```python
from build123d import *

# Parameters (mm, degrees)
F0_W     = 10
F0_H     = 4
F0_R     = 0.4
F0_R_2   = 0.425
F0_R_3   = 0.45
F0_R_4   = 0.475
F0_R_5   = 0.5
F1_DEPTH = 3
F2_R     = 1


with BuildPart() as f1:
    # F0 (on Front) → F1 (new body)
    with BuildSketch(Plane.XZ):
        Rectangle(F0_W, F0_H)
        with Locations((-3.333333, 0)):
            Circle(F0_R, mode=Mode.SUBTRACT)
        with Locations((-1.666667, 0)):
            Circle(F0_R_2, mode=Mode.SUBTRACT)
        Circle(F0_R_3, mode=Mode.SUBTRACT)
        with Locations((1.666667, 0)):
            Circle(F0_R_4, mode=Mode.SUBTRACT)
        with Locations((3.333333, 0)):
            Circle(F0_R_5, mode=Mode.SUBTRACT)
    extrude(amount=F1_DEPTH)

    # F2
    f2_edges = [f1.edges().sort_by_distance(p)[0] for p in [
        (5, -1.5, 2),
        (5, -1.5, -2),
    ]]
    fillet(f2_edges, radius=F2_R)


solid = f1.part
```
Geometry check sheet. Reference: the model listing, model coordinates, mm. Coordinates: 2 decimals unless noted, no trailing zeros. Write each loop counter-clockwise with the first axis right and the second up, starting at its lowest first coordinate (ties: lowest second). Pieces come first, ordered by that corner, then holes. Notation, with made-up numbers: M 41.25,16.25 L 89.25,16.25 A29 ccw 89.25,42.25 Z; hole C -31.75,22.25 d6. An arc over 180 degrees is marked long. Use one line per item in the form item = value. Start each with the question number.
1) Section check A-A on z = 0. Enter the section's corners in (x, y).
2) Section check D-D on x = 1.5. Enter the section's corners in (y, z).
3) Section check B-B on x = 0. Enter the section's corners in (y, z).
4) Release check for a two-part mould opening along Z. For faces 1 (the cylindrical face through (4.699, -1.521, -1.715)), 2 (the flat face through (-1, -1, 2)), 3 (the flat face through (0, -3, 1)), 4 (the cylindrical face through (3.795, -1.479, -0.192)) record: pulls with the +Z half, pulls with the -Z half, needs draft (parallel to the pull), parting line crosses it, or undercut.
5) Thickness scan on probe 1 along Z at (x, y) = (0, -0.7); probe 2 along X at (y, z) = (-0.65, -0.15); probe 3 along Z at (x, y) = (2, -2). Record the ranges inside material, lowest first. Write a range as from..to.
6) Section check C-C on y = -2.5. Enter the section's corners in (x, z) (3 decimals), and give its area (3 significant figures).
Responses:
q1.outline = M -5,-3 L -3.73,-3 L -3.73,0 L -5,0 Z; M -2.93,-3 L -2.09,-3 L -2.09,0 L -2.93,0 Z; M -1.24,-3 L -0.45,-3 L -0.45,0 L -1.24,0 Z; M 0.45,-3 L 1.19,-3 L 1.19,0 L 0.45,0 Z; M 2.14,-3 L 2.83,-3 L 2.83,0 L 2.14,0 Z; M 3.83,-3 L 5,-3 L 5,0 L 3.83,0 Z
q2.outline = M -3,-2 L 0,-2 L 0,-0.44 L -3,-0.44 Z; M -3,0.44 L 0,0.44 L 0,2 L -3,2 Z
q3.outline = M -3,-2 L 0,-2 L 0,-0.45 L -3,-0.45 Z; M -3,0.45 L 0,0.45 L 0,2 L -3,2 Z
q4.face_1 = pulls with the -Z half
q4.face_2 = pulls with the +Z half
q4.face_3 = needs draft
q4.face_4 = undercut
q5.probe_1 = -2..-0.45, 0.45..2
q5.probe_2 = -5..-3.7, -2.96..-2.06, -1.27..-0.42, 0.42..1.22, 2.12..2.86, 3.81..5
q5.probe_3 = -2..-0.34, 0.34..2
q6.outline = M -5,-2 L 4,-2 A1 ccw 5,-1 L 5,1 A1 ccw 4,2 L -5,2 Z; hole C -3.333,0 d0.8; hole C -1.667,0 d0.85; hole C 0,0 d0.9; hole C 1.667,0 d0.95; hole C 3.333,0 d1
q6.area = 36.4 mm2
